Check sheet for the modelled part. Datum: model origin and axes. Units: mm. Round coordinates to 2 decimals unless told otherwise and drop trailing zeros. Write each loop counter-clockwise with the first axis right and the second up, starting at its lowest first coordinate (ties: lowest second). Pieces come first, ordered by that corner, then holes.
from build123d import *

# Parameters (mm, degrees)
F0_W     = 63.5
F0_H     = 25.4
F1_DEPTH = 12.7
F3_D     = 12.7


# Not quite as in the source:
# - a length typed as a fraction of an inch, garbled in the dataset ("3 / 203.2 mm" for 3/8 in), is restored


with BuildPart() as f1:
    # F0 (on Front) → F1 (new body)
    with BuildSketch(Plane.XZ):
        Rectangle(F0_W, F0_H)
    extrude(amount=F1_DEPTH)

    # F3 (through all)
    with Locations(Plane.XZ.offset(12.7)):
        with Locations((-19.05, 0), (19.05, 0)):
            Hole(F3_D / 2)


solid = f1.part
1. Release check for a two-part mould opening along Z. For faces 1 (the flat face through (0, -6, -12.7)), 2 (the flat face through (0, 0, 0)), 3 (the flat face through (0, -6, 12.7)), 4 (the cylindrical face through (-24.916, -6.261, -2.432)) record: released by +Z, released by -Z, zero draft, split by the parting line, or undercut.
2. Sectioned sample at C-C, the plane z = 5.5. Enter the section's corners in (x, y).
3. Sectioned sample at A-A, the plane x = -19.05. Enter the section's corners in (y, z).
4. Sectioned sample at B-B, the plane y = -1.25. Enter the section's corners in (x, z).
5. Sectioned sample at D-D, the plane z = -3.75. Enter the section's corners in (x, y), plus the area to 3 significant figures.
6. Scan lines: line 1 along X through (y, z) = (-6.75, 0.25); line 2 along Z through (x, y) = (-19.05, -8); line 3 along X through (y, z) = (-2, 2.25). Record each from-to range of solid material in increasing order.
Computed values:
1. face 1: released by -Z
1. face 2: zero draft
1. face 3: released by +Z
1. face 4: undercut
2. outline: (-31.75, -12.7) - (-22.22, -12.7) - (-22.22, 0) - (-31.75, 0) - close; (-15.88, -12.7) - (15.88, -12.7) - (15.88, 0) - (-15.88, 0) - close; (22.22, -12.7) - (31.75, -12.7) - (31.75, 0) - (22.22, 0) - close
3. outline: (-12.7, -12.7) - (0, -12.7) - (0, -6.35) - (-12.7, -6.35) - close; (-12.7, 6.35) - (0, 6.35) - (0, 12.7) - (-12.7, 12.7) - close
4. outline: (-31.75, -12.7) - (31.75, -12.7) - (31.75, 12.7) - (-31.75, 12.7) - close; hole circle Ø12.7 at (-19.05, 0); hole circle Ø12.7 at (19.05, 0)
5. outline: (-31.75, -12.7) - (-24.17, -12.7) - (-24.17, 0) - (-31.75, 0) - close; (-13.93, -12.7) - (13.93, -12.7) - (13.93, 0) - (-13.93, 0) - close; (24.17, -12.7) - (31.75, -12.7) - (31.75, 0) - (24.17, 0) - close
5. area: 546 mm2
6. line 1: x = -31.75 to -25.4, -12.7 to 12.7, 25.4 to 31.75
6. line 2: z = -12.7 to -6.35, 6.35 to 12.7
6. line 3: x = -31.75 to -24.99, -13.11 to 13.11, 24.99 to 31.75
